```python
from build123d import *

# Parameters (mm, degrees)
CROQUIS1_W              = 53
CROQUIS1_H              = 44
CROQUIS1_R              = 1.75
SALIENTE_EXTRUIR1_DEPTH = 6.5
CROQUIS3_W              = 43
CROQUIS3_H              = 1.75
SALIENTE_EXTRUIR2_DEPTH = 5
CROQUIS4_W              = 43
CROQUIS4_H              = 1.75
SALIENTE_EXTRUIR3_DEPTH = 2.5
CROQUIS5_W              = 53
CROQUIS5_H              = 8
CORTAR_EXTRUIR2_DEPTH   = 1.5
CROQUIS8_W              = 2
CROQUIS8_H              = 8
SALIENTE_EXTRUIR6_DEPTH = 3
SALIENTE_EXTRUIR7_DEPTH = 8
CORTAR_EXTRUIR3_DEPTH   = 3


with BuildPart() as part:
    # Croquis1 → Saliente-Extruir1 (new body)
    with BuildSketch(Plane.XY):
        Rectangle(CROQUIS1_W, CROQUIS1_H)
        with Locations(Location((21.5, 0, 0), (0, 0, 180))):
            Circle(CROQUIS1_R, mode=Mode.SUBTRACT)
    extrude(amount=SALIENTE_EXTRUIR1_DEPTH)

    # Croquis3 → Saliente-Extruir2 (add)
    with BuildSketch(Plane(origin=(0, 0, 0), x_dir=(-1, 0, 0), z_dir=(0, 0, -1))):
        with Locations((5, -21.125)):
            Rectangle(CROQUIS3_W, CROQUIS3_H)
        with Locations((5, 21.125)):
            Rectangle(CROQUIS3_W, CROQUIS3_H)
    extrude(amount=SALIENTE_EXTRUIR2_DEPTH)

    # Croquis4 → Saliente-Extruir3 (add)
    with BuildSketch(Plane(origin=(0, 0, -5), x_dir=(-1, 0, 0), z_dir=(0, 0, -1))):
        with Locations((5, -19.375)):
            Rectangle(CROQUIS4_W, CROQUIS4_H)
        with Locations((5, 19.375)):
            Rectangle(CROQUIS4_W, CROQUIS4_H)
    extrude(amount=-SALIENTE_EXTRUIR3_DEPTH)

    # Croquis5 → Cortar-Extruir2 (cut)
    with BuildSketch(Plane(origin=(0, 0, 0), x_dir=(-1, 0, 0), z_dir=(0, 0, -1))):
        Rectangle(CROQUIS5_W, CROQUIS5_H)
    extrude(amount=-CORTAR_EXTRUIR2_DEPTH, mode=Mode.SUBTRACT)

    # Croquis8 → Saliente-Extruir6 (add)
    with BuildSketch(Plane(origin=(0, 0, 1.5), x_dir=(-1, 0, 0), z_dir=(0, 0, -1))):
        with Locations((25.5, 0)):
            Rectangle(CROQUIS8_W, CROQUIS8_H)
    extrude(amount=SALIENTE_EXTRUIR6_DEPTH)

    # Croquis9 → Saliente-Extruir7 (add)
    with BuildSketch(Plane.XZ.offset(-4)):
        Polygon((-24.5, 1.5), (-18.5, 1.5), (-24.5, 0.75), align=None)
    extrude(amount=SALIENTE_EXTRUIR7_DEPTH)

    # Croquis10 → Cortar-Extruir3 (cut)
    with BuildSketch(Plane.XY.offset(6.5)):
        Polygon((21.5, -3.5), (24.531088913, -1.75), (24.531088913, 1.75), (21.5, 3.5), (18.468911087, 1.75), (18.468911087, -1.75), align=None)
    extrude(amount=-CORTAR_EXTRUIR3_DEPTH, mode=Mode.SUBTRACT)


solid = part.part
```
Input: part model. Units: mm. Frame: model coordinates. A direction names the side the tool comes from. Give positions to 0.01 mm unless a question says otherwise; leave off trailing zeros. Write each loop counter-clockwise with the first axis right and the second up, starting at its lowest first coordinate (ties: lowest second). Pieces come first, ordered by that corner, then holes. Notation, with made-up numbers: (57.25, 17.25) - (62.25, 17.25) arc R19 cw to (62.25, 51.25) - close; hole circle Ø7 at (71, 62). An arc over 180 degrees is marked (long way). Write item = value, one per line. Start each with the question number.
1. Mould query, pull axis Z, two halves, no side actions, for faces 1 (the flat face through (0, 0, 6.5)), 2 (the flat face through (-25, 0, -1.5)), 3 (the flat face through (-5, 20.25, -1)), 4 (the flat face through (19.96, -2.61, 5.02)). Classes: released by +Z, released by -Z, zero draft, split by the parting line, or undercut.
2. Section query B-B, the plane x = 9.5. Output: boundary loops of the cut face in (y, z), then the cut area to 3 significant figures.
3. Section query C-C, the plane y = 10. Output: boundary loops of the cut face in (x, z), then the cut area to 4 significant figures.
4. Ray query, L1, parallel to Z at x = -1, y = -20; L2, parallel to Y at x = 21.5, z = 2.65; L3, parallel to Z at x = 19.5, y = -13.5. Return the intervals inside material, ascending.
5. Access query for faces 5 (the flat face through (-26.5, 0, 2)), 6 (the flat face through (20, -2, 3.5)), 7 (the flat face through (4, 0, 1.5)), 8 (the flat face through (-5, -20, -5)), 9 (the flat face through (-5, 18.5, -4)). Directions: +Z, -Z, +X, -X, +Y, -Y. A direction counts if a zero-diameter tool reaches every point of the face in a straight line with its end or side. Return the directions, or none.
6. First-contact query: pin 1 Ø1 at (y, z) = (21, -3.5) entering from +X; pin 2 Ø2 at (x, y) = (-25.5, 2) entering from -Z; pin 3 Ø4 at (x, y) = (9.5, 1.5) entering from -Z; pin 4 Ø2 at (y, z) = (2, -3.5) entering from -X. Flat tips, straight axial feed; report the tip coordinate or a pass-through.
7. Section query A-A, the plane y = 0. Output: boundary loops of the cut face in (x, z).
8. Section query D-D, the plane x = -22. Output: boundary loops of the cut face in (y, z).
Check sheet entries:
q1.face_1 = released by +Z
q1.face_2 = released by -Z
q1.face_3 = undercut
q1.face_4 = zero draft
q2.outline = (-22, -5) - (-18.5, -5) - (-18.5, -2.5) - (-20.25, -2.5) - (-20.25, 0) - (-4, 0) - (-4, 1.5) - (4, 1.5) - (4, 0) - (20.25, 0) - (20.25, -2.5) - (18.5, -2.5) - (18.5, -5) - (22, -5) - (22, 6.5) - (-22, 6.5) - close
q2.area = 300 mm2
q3.outline = (-26.5, 0) - (26.5, 0) - (26.5, 6.5) - (-26.5, 6.5) - close
q3.area = 344.5 mm2
q4.L1 = -5 to -2.5, 0 to 6.5
q4.L2 = -22 to -1.75, 1.75 to 22
q4.L3 = 0 to 6.5
q5.face_5 = +Z, -Z, -X, +Y, -Y
q5.face_6 = +Z
q5.face_7 = -Z, +X
q5.face_8 = -Z, +X, -X, +Y, -Y
q5.face_9 = -Z, +X, -X
q6.pin_1 = 16.5
q6.pin_2 = -1.5
q6.pin_3 = 1.5
q6.pin_4 = through
q7.outline = (-26.5, -1.5) - (-24.5, -1.5) - (-24.5, 0.75) - (-18.5, 1.5) - (19.75, 1.5) - (19.75, 3.5) - (18.47, 3.5) - (18.47, 6.5) - (-26.5, 6.5) - close; (23.25, 1.5) - (26.5, 1.5) - (26.5, 6.5) - (24.53, 6.5) - (24.53, 3.5) - (23.25, 3.5) - close
q8.outline = (-22, -5) - (-18.5, -5) - (-18.5, -2.5) - (-20.25, -2.5) - (-20.25, 0) - (-4, 0) - (-4, 1.06) - (4, 1.06) - (4, 0) - (20.25, 0) - (20.25, -2.5) - (18.5, -2.5) - (18.5, -5) - (22, -5) - (22, 6.5) - (-22, 6.5) - close
